from build123d import *

# Parameters (mm, degrees)
F0_R     = 2.5
F0_R_2   = 1.25
F1_DEPTH = 10
F0_R_3   = 5
F2_DEPTH = 2
F3_R     = 1.5
F4_SIZE  = 1


with BuildPart() as f1:
    # F0 (on Front) → F1 (new body)
    with BuildSketch(Plane.XZ):
        Circle(F0_R)
        Circle(F0_R_2, mode=Mode.SUBTRACT)
    extrude(amount=F1_DEPTH)

    # F0 (on Front) → F2 (join)
    with BuildSketch(Plane.XZ):
        Circle(F0_R_3)
        Circle(F0_R, mode=Mode.SUBTRACT)
    extrude(amount=F2_DEPTH)

    # F3
    f3_edges = [f1.edges().sort_by_distance(p)[0] for p in [
        (-5, 0, 0),
    ]]
    fillet(f3_edges, radius=F3_R)

    # F4
    f4_edges = [f1.edges().sort_by_distance(p)[0] for p in [
        (-1.25, 0, 0),
    ]]
    chamfer(f4_edges, length=F4_SIZE)


solid = f1.part
Source: CAD feature listing. Evaluate the final solid. Frame: model axes, mm. A direction names the side the tool comes from. Round coordinates to 2 decimals unless told otherwise and drop trailing zeros. Loops run counter-clockwise (first coordinate to the right, second up) from the corner with the lowest first, then second, coordinate; pieces in that order, holes last. Notation, with made-up numbers: (63, -34) -> (101, -34) arc R12 cw to (101, -27) -> close; hole circle Ø10 at (-12.5, 74). An arc over 180 degrees is marked (long way). Answer as a JSON object with one key per item and string values. Group by question number.
Q1. Access query for faces 1 (the cylindrical face through (-1.08, -1.75, -4.88)), 2 (the cylindrical face through (-0.54, -5.94, -2.44)). Directions: +Z, -Z, +X, -X, +Y, -Y. A direction counts if a zero-diameter tool reaches every point of the face in a straight line with its end or side. Return the directions, or none.
Q2. Contact query for flat-ended pins moving along their axis: P1, Ø1.5, axis at x = 3, z = -0.5, coming from the -Y side; P2, Ø1, axis at x = 2, z = 3.5, coming from the -Y side; P3, Ø1.5, axis at y = -5, z = -3.5, coming from the -X side; P4, Ø1, axis at x = -2, y = -1, coming from the +Z side. Output: stop coordinate, or through.
Q3. Ray query, line 1 (Z direction, x = 0, y = -7.75); line 2 (Y direction, x = 2.75, z = -0.75); line 3 (Z direction, x = -1, y = -7.5). Return the intervals inside material, ascending. Write a range as from..to.
Q4. Section query A-A (z = 0). Output: boundary loops of the cut face in (x, y).
Q5. Section query C-C (y = -3.25). Output: boundary loops of the cut face in (x, z), plus the area to 3 significant figures.
Q6. Section query B-B (x = 0). Output: boundary loops of the cut face in (y, z).
Completed:
{
 "1": {"face 1": "+Y, -Y", "face 2": "-Y"},
 "2": {"P1": "y = -10", "P2": "y = -2", "P3": "through", "P4": "z = 4.73"},
 "3": {"line 1": "-2.5..-1.25, 1.25..2.5", "line 2": "-2..0", "line 3": "-2.29..-0.75, 0.75..2.29"},
 "4": {"outline": "(-5, -2) -> (-2.5, -2) -> (-2.5, -10) -> (-1.25, -10) -> (-1.25, -1) -> (-2.25, 0) -> (-3.5, 0) arc R1.5 ccw to (-5, -1.5) -> close; (1.25, -10) -> (2.5, -10) -> (2.5, -2) -> (5, -2) -> (5, -1.5) arc R1.5 ccw to (3.5, 0) -> (2.25, 0) -> (1.25, -1) -> close"},
 "5": {"outline": "circle Ø5 at (0, 0); hole circle Ø2.5 at (0, 0)", "area": "14.7 mm²"},
 "6": {"outline": "(-10, -2.5) -> (-2, -2.5) -> (-2, -5) -> (-1.5, -5) arc R1.5 ccw to (0, -3.5) -> (0, -2.25) -> (-1, -1.25) -> (-10, -1.25) -> close; (-10, 1.25) -> (-1, 1.25) -> (0, 2.25) -> (0, 3.5) arc R1.5 ccw to (-1.5, 5) -> (-2, 5) -> (-2, 2.5) -> (-10, 2.5) -> close"}
}
